Part model, mm, in its own coordinate system. Face numbers are marked on the shaded views. A direction names the side the tool comes from. Give positions to 0.01 mm unless a question says otherwise; leave off trailing zeros. Order: outer loops, then holes, each group sorted by start corner. A loop starts at its lowest first (then second) coordinate and runs counter-clockwise, first axis right, second up. Notation, with made-up numbers: (57, 64) -> (71, 64) arc R10 cw to (71, 82) -> close; hole circle Ø11 at (5, -25). An arc over 180 degrees is marked (long way). Write item = value, one per line. Start each with the question number.
Item 1: Drill centre lines: line 1 along Y through (x, z) = (0, -23); line 2 along Y through (x, z) = (119, 30.5); line 3 along Y through (x, z) = (23, 41.5). Where is each one in solid material? Low to high.
Item 2: Pull direction X, two halves, no side cores. Call the marked faces 1, 2 and 3: +X half, -X half, draft (parallel to the pull), parting line (faces both ways), or undercut.
Item 3: Flat gauge pins, fed straight in: P1, Ø1.8, axis at x = -115, y = -61, coming from the +Z side; P2, Ø6.5, axis at x = 114.5, y = -69, coming from the -Z side; P3, Ø5, axis at x = 64, z = 43, coming from the -Y side; P4, Ø17.5, axis at x = 68.5, z = 0, coming from the +Y side. Where does each tip first touch, or does it go through?
Item 4: Band-saw the part on C-C on y = 10. Write the cut outline in (x, z).
Item 5: Band-saw the part on A-A on x = 0. Write the cut outline in (y, z), plus the area to 3 significant figures.
Item 6: Band-saw the part on B-B on z = 25. Write the cut outline in (x, y).
Item 7: Tool access for the marked faces 4, 5 and 6: list every direction of +Z, -Z, +X, -X, +Y, -Y with a clear straight run to the whole face (end or side of a thin tool).
Item 8: Band-saw the part on D-D on y = -45. Write the cut outline in (x, z).
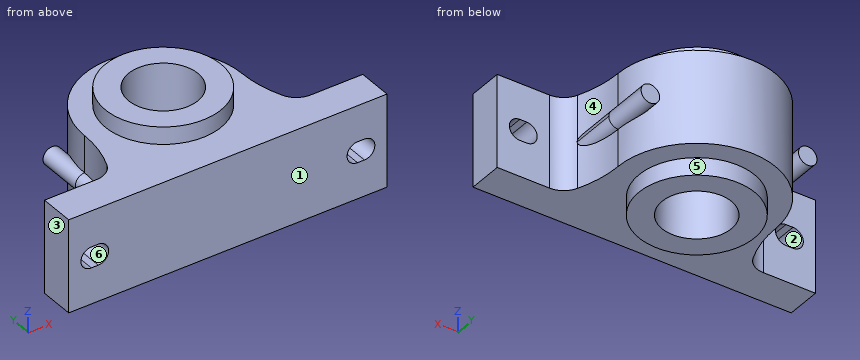
```python
from build123d import *

# Parameters (mm, degrees)
SKETCH1_R                = 30
BOSS_EXTRUDE1_DEPTH      = 40
SKETCH2_R                = 50
SKETCH2_R_2              = 30
BOSS_EXTRUDE2_DEPTH      = 55
CUT_EXTRUDE1_DEPTH       = 110
SKETCH5_R                = 8
BOSS_EXTRUDE3_DEPTH      = 40
BOSS_EXTRUDE3_DEPTH_BACK = 60


with BuildPart() as part:
    # Sketch1 → Boss-Extrude1 (new body, symmetric)
    with BuildSketch(Plane.XY):
        with BuildLine():
            Line((137.5, -80), (-137.5, -80))
            Line((-137.5, -80), (-137.5, -50))
            Line((-137.5, -50), (-92.5, -50))
            ThreePointArc((-92.5, -50), (-82.586036695, -47.018171653), (-75.961854895, -39.062156056))
            ThreePointArc((-75.961854895, -39.062156056), (-70.010718453, -19.932656428), (-68, 0))
            ThreePointArc((-68, 0), (0, 68), (68, 0))
            ThreePointArc((68, 0), (70.010718453, -19.932656428), (75.961854895, -39.062156056))
            ThreePointArc((75.961854895, -39.062156056), (82.586036695, -47.018171653), (92.5, -50))
            Line((92.5, -50), (137.5, -50))
            Line((137.5, -50), (137.5, -80))
        make_face()
        Circle(SKETCH1_R, mode=Mode.SUBTRACT)
    extrude(amount=BOSS_EXTRUDE1_DEPTH, both=True)

    # Sketch2 → Boss-Extrude2 (add, symmetric)
    with BuildSketch(Plane.XY):
        Circle(SKETCH2_R)
        Circle(SKETCH2_R_2, mode=Mode.SUBTRACT)
    extrude(amount=BOSS_EXTRUDE2_DEPTH, both=True)

    # Sketch3 → Cut-Extrude1 (cut)
    with BuildSketch(Plane(origin=(0, 0, 0), x_dir=(1, 0, 0), z_dir=(0, 1, 0))):
        with BuildLine():
            Line((-118, 9), (-112, 9))
            ThreePointArc((-112, 9), (-103, 0), (-112, -9))
            Line((-112, -9), (-118, -9))
            ThreePointArc((-118, -9), (-127, 0), (-118, 9))
        make_face()
        with BuildLine():
            Line((118, 9), (112, 9))
            ThreePointArc((112, 9), (103, 0), (112, -9))
            Line((112, -9), (118, -9))
            ThreePointArc((118, -9), (127, 0), (118, 9))
        make_face()
    extrude(amount=-CUT_EXTRUDE1_DEPTH, mode=Mode.SUBTRACT)

    # Sketch5 → Boss-Extrude3 (add, two sides)
    with BuildSketch(Plane(origin=(0, 0, 0), x_dir=(1, 0, 0), z_dir=(0, 1, 0))) as boss_extrude3_sk:
        with Locations((-68, 0)):
            Circle(SKETCH5_R)
        with Locations((68, 0)):
            Circle(SKETCH5_R)
    extrude(amount=BOSS_EXTRUDE3_DEPTH)
    extrude(boss_extrude3_sk.sketch, amount=-BOSS_EXTRUDE3_DEPTH_BACK)


solid = part.part
```
Values found:
q1.line_1 = -80 to -30, 30 to 68
q1.line_2 = -80 to -50
q1.line_3 = -44.4 to -19.26, 19.26 to 44.4
q2.face_1 = draft
q2.face_2 = undercut
q2.face_3 = -X half
q3.P1 = 40
q3.P2 = -40
q3.P3 = through
q3.P4 = 40
q4.outline = (-67.26, -40) -> (-48.99, -40) -> (-48.99, -55) -> (-28.28, -55) -> (-28.28, 55) -> (-48.99, 55) -> (-48.99, 40) -> (-67.26, 40) -> (-67.26, 7.97) arc R8 ccw (long way) to (-67.26, -7.97) -> close; (28.28, -55) -> (48.99, -55) -> (48.99, -40) -> (67.26, -40) -> (67.26, -7.97) arc R8 ccw (long way) to (67.26, 7.97) -> (67.26, 40) -> (48.99, 40) -> (48.99, 55) -> (28.28, 55) -> close
q5.outline = (-80, -40) -> (-50, -40) -> (-50, -55) -> (-30, -55) -> (-30, 55) -> (-50, 55) -> (-50, 40) -> (-80, 40) -> close; (30, -55) -> (50, -55) -> (50, -40) -> (68, -40) -> (68, 40) -> (50, 40) -> (50, 55) -> (30, 55) -> close
q5.area = 8,240 mm^2
q6.outline = (-137.5, -80) -> (137.5, -80) -> (137.5, -50) -> (92.5, -50) arc R17.97 cw to (75.96, -39.06) arc R99.8 cw to (68, 0) arc R68 ccw to (-68, 0) arc R99.8 cw to (-75.96, -39.06) arc R17.97 cw to (-92.5, -50) -> (-137.5, -50) -> close; hole circle Ø60 at (0, 0)
q7.face_4 = +Z, +X, +Y
q7.face_5 = -Z
q7.face_6 = +Y, -Y
q8.outline = (-80.06, -40) -> (-21.79, -40) -> (-21.79, -55) -> (21.79, -55) -> (21.79, -40) -> (80.06, -40) -> (80.06, 40) -> (21.79, 40) -> (21.79, 55) -> (-21.79, 55) -> (-21.79, 40) -> (-80.06, 40) -> close
